Source: CAD feature listing. Evaluate the final solid. Frame: model axes, mm. Face numbers are marked on the shaded views. A direction names the side the tool comes from. Coordinates: 2 decimals unless noted, no trailing zeros. Order: outer loops, then holes, each group sorted by start corner. A loop starts at its lowest first (then second) coordinate and runs counter-clockwise, first axis right, second up. Notation, with made-up numbers: (-9.5, 19) -> (43.5, 19) arc R10 cw to (43.5, 24) -> close; hole circle Ø11 at (84, 39.5). An arc over 180 degrees is marked (long way). Write each question's results on one line, items separated by ' | '. Start each with the question number.
from build123d import *

# Parameters (mm, degrees)
SALIENTE_EXTRUIR1_DEPTH = 80
CROQUIS2_W              = 40
CROQUIS2_H              = 40
CORTAR_EXTRUIR1_DEPTH   = 80
CROQUIS3_W              = 40
CROQUIS3_H              = 40
CORTAR_EXTRUIR2_DEPTH   = 80
REDONDEO1_R             = 2
CROQUIS4_W              = 20
CROQUIS4_H              = 20
CORTAR_EXTRUIR3_DEPTH   = 80
CROQUIS5_W              = 20
CROQUIS5_H              = 20
CORTAR_EXTRUIR4_DEPTH   = 50
CROQUIS6_W              = 20
CROQUIS6_H              = 20
CORTAR_EXTRUIR5_DEPTH   = 50


with BuildPart() as part:
    # Croquis1 → Saliente-Extruir1 (new body)
    with BuildSketch(Plane(origin=(0, 0, 0), x_dir=(1, 0, 0), z_dir=(0, 1, 0))):
        Polygon((0, 80), (0, 0), (80, 0), (80, 40), (40, 40), (40, 80), align=None)
    extrude(amount=SALIENTE_EXTRUIR1_DEPTH)

    # Croquis2 → Cortar-Extruir1 (cut)
    with BuildSketch(Plane.XY):
        with Locations((60, 60)):
            Rectangle(CROQUIS2_W, CROQUIS2_H)
    extrude(amount=-CORTAR_EXTRUIR1_DEPTH, mode=Mode.SUBTRACT)

    # Croquis3 → Cortar-Extruir2 (cut)
    with BuildSketch(Plane(origin=(40, 0, 0), x_dir=(0, 0, -1), z_dir=(1, 0, 0))):
        with Locations((60, 60)):
            Rectangle(CROQUIS3_W, CROQUIS3_H)
    extrude(amount=-CORTAR_EXTRUIR2_DEPTH, mode=Mode.SUBTRACT)

    # Redondeo1
    # the kernel refuses this fillet: 2 mm, written as the material it takes off along each edge
    with BuildSketch(Plane(origin=(0, -5, 0), x_dir=(0, 0, -1), z_dir=(0, 1, 0))) as redondeo1_piece_1:
        with BuildLine():
            CenterArc((REDONDEO1_R, -REDONDEO1_R), REDONDEO1_R, 90, 90)
            Line((0, -REDONDEO1_R), (0, 0))
            Line((0, 0), (REDONDEO1_R, 0))
        make_face()
    extrude(amount=90, mode=Mode.SUBTRACT)
    with BuildSketch(Plane(origin=(80, -5, -40), x_dir=(0, 0, 1), z_dir=(0, 1, 0)), Plane(origin=(80, -5, 0), x_dir=(-1, 0, 0), z_dir=(0, 1, 0)), Plane(origin=(40, 45, -80), x_dir=(-1, 0, 0), z_dir=(0, -1, 0))) as redondeo1_piece_2:
        with BuildLine():
            CenterArc((REDONDEO1_R, -REDONDEO1_R), REDONDEO1_R, 90, 90)
            Line((0, -REDONDEO1_R), (0, 0))
            Line((0, 0), (REDONDEO1_R, 0))
        make_face()
    extrude(amount=50, mode=Mode.SUBTRACT)
    with BuildSketch(Plane(origin=(40, 85, 0), x_dir=(-1, 0, 0), z_dir=(0, -1, 0))) as redondeo1_piece_3:
        with BuildLine():
            CenterArc((REDONDEO1_R, REDONDEO1_R), REDONDEO1_R, 180, 90)
            Line((0, REDONDEO1_R), (0, 0))
            Line((0, 0), (REDONDEO1_R, 0))
        make_face()
    extrude(amount=45, mode=Mode.SUBTRACT)
    with BuildSketch(Plane(origin=(0, -5, -80), x_dir=(0, 0, 1), z_dir=(0, 1, 0))) as redondeo1_piece_4:
        with BuildLine():
            CenterArc((REDONDEO1_R, REDONDEO1_R), REDONDEO1_R, 180, 90)
            Line((0, REDONDEO1_R), (0, 0))
            Line((0, 0), (REDONDEO1_R, 0))
        make_face()
    extrude(amount=50, mode=Mode.SUBTRACT)
    with BuildSketch(Plane(origin=(0, 85, -40), x_dir=(0, 0, 1), z_dir=(0, -1, 0)), Plane(origin=(40, 85, -40), x_dir=(-1, 0, 0), z_dir=(0, -1, 0))) as redondeo1_piece_5:
        with BuildLine():
            CenterArc((REDONDEO1_R, -REDONDEO1_R), REDONDEO1_R, 90, 90)
            Line((0, -REDONDEO1_R), (0, 0))
            Line((0, 0), (REDONDEO1_R, 0))
        make_face()
    extrude(amount=45, mode=Mode.SUBTRACT)

    # Croquis4 → Cortar-Extruir3 (cut)
    with BuildSketch(Plane(origin=(0, 80, 0), x_dir=(1, 0, 0), z_dir=(0, 1, 0))):
        with Locations((20, 20)):
            Rectangle(CROQUIS4_W, CROQUIS4_H)
    extrude(amount=-CORTAR_EXTRUIR3_DEPTH, mode=Mode.SUBTRACT)

    # Croquis5 → Cortar-Extruir4 (cut)
    with BuildSketch(Plane(origin=(0, 0, -80), x_dir=(-1, 0, 0), z_dir=(0, 0, -1))):
        with Locations((-20, 20)):
            Rectangle(CROQUIS5_W, CROQUIS5_H)
    extrude(amount=-CORTAR_EXTRUIR4_DEPTH, mode=Mode.SUBTRACT)

    # Croquis6 → Cortar-Extruir5 (cut)
    with BuildSketch(Plane(origin=(80, 0, 0), x_dir=(0, 0, -1), z_dir=(1, 0, 0))):
        with Locations((20, 20)):
            Rectangle(CROQUIS6_W, CROQUIS6_H)
    extrude(amount=-CORTAR_EXTRUIR5_DEPTH, mode=Mode.SUBTRACT)


solid = part.part
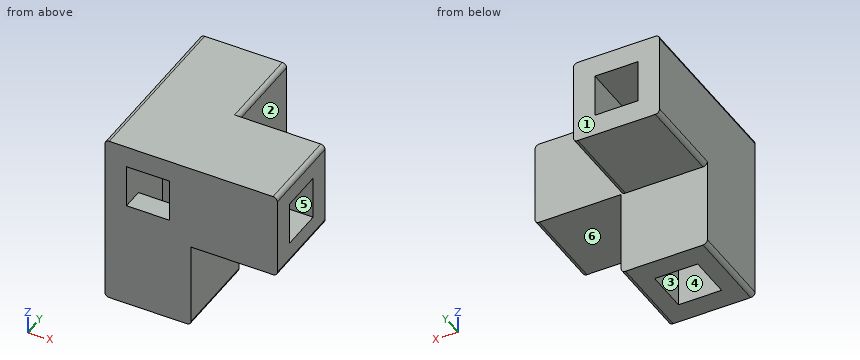
(1) Draft query along X for the marked faces 1, 2 and 3. Return one class per face: released by +X, released by -X, zero draft, split by the parting line, or undercut.
(2) Section A-A on y = 18.5. Return the cut outline in (x, z).
(3) First-contact query: P1, Ø22, axis at x = 15.5, z = -53, coming from the +Y side; P2, Ø19, axis at x = 52, y = 10.5, coming from the -Z side; P3, Ø11, axis at y = 65.5, z = -22, coming from the +X side; P4, Ø5, axis at y = 29, z = -54.5, coming from the -X side. Flat tips, straight axial feed; report the tip coordinate or a pass-through.
(4) Section D-D on z = -21.5. Return the cut outline in (x, y).
(5) Section B-B on z = -66. Return the cut outline in (x, y).
(6) Line query: L1, parallel to Z at x = 32.5, y = 28.5; L2, parallel to Y at x = 28.5, z = -38; L3, parallel to Z at x = 60, y = 23.5. Output: solid intervals per line, ascending.
(7) Reachability of the marked faces 4, 5 and 6 from +Z, -Z, +X, -X, +Y, -Y: full face, straight path, thin tool, end or side. Return the list, or none.
(8) Section C-C on x = 11.5. Return the cut outline in (y, z), then the cut area to 3 significant figures.
Results list:
1) face 1: zero draft | face 2: released by +X | face 3: undercut
2) outline: (0, -78) arc R2 ccw to (2, -80) -> (10, -80) -> (10, -10) -> (80, -10) -> (80, -2) arc R2 ccw to (78, 0) -> (2, 0) arc R2 ccw to (0, -2) -> close; (30, -80) -> (38, -80) arc R2 ccw to (40, -78) -> (40, -40) -> (78, -40) arc R2 ccw to (80, -38) -> (80, -30) -> (30, -30) -> close
3) P1: stops at y = 40 | P2: stops at z = -40 | P3: stops at x = 40 | P4: stops at x = 0
4) outline: (0, 0) -> (10, 0) -> (10, 80) -> (0, 80) -> close; (30, 0) -> (80, 0) -> (80, 10) -> (30, 10) -> close; (30, 30) -> (80, 30) -> (80, 40) -> (40, 40) -> (40, 80) -> (30, 80) -> close
5) outline: (0, 0) -> (40, 0) -> (40, 40) -> (0, 40) -> close; hole (10, 10) -> (30, 10) -> (30, 30) -> (10, 30) -> close
6) L1: z = -80 to -30, -10 to 0 | L2: y = 0 to 10, 30 to 80 | L3: z = -40 to -30, -10 to 0
7) face 4: -Z | face 5: +X | face 6: -Z, +X, +Y, -Y
8) outline: (0, -80) -> (10, -80) -> (10, -30) -> (0, -30) -> close; (0, -10) -> (80, -10) -> (80, 0) -> (0, 0) -> close; (30, -80) -> (40, -80) -> (40, -40) -> (80, -40) -> (80, -30) -> (30, -30) -> close | area: 2,200 mm²
